The listing builds one solid part. Answer for the finished solid, in the listing's coordinates (mm). A direction names the side the tool comes from. Coordinates: 2 decimals unless noted, no trailing zeros. Loops run counter-clockwise (first coordinate to the right, second up) from the corner with the lowest first, then second, coordinate; pieces in that order, holes last. Notation, with made-up numbers: (-20.5, -37) -> (-10.5, -37) arc R21 cw to (-10.5, -5) -> close; hole circle Ø4 at (67, 53.25). An arc over 180 degrees is marked (long way). Answer in a Markdown table with one row per item.
```python
from build123d import *

# Parameters (mm, degrees)
F1_DEPTH  = 50.8
F2_T      = -1.5875
F4_DEPTH  = 1.5875
F5_W      = 15.875
F5_H      = 12.7
F6_DEPTH  = 1.5875
F7_W      = 1.5875
F7_H      = 12.7
F8_DEPTH  = 15.875
F10_D     = 6.7564
F11_W     = 15.875
F11_H     = 12.7
F12_DEPTH = 1.5875
F13_W     = 1.5875
F13_H     = 12.7
F14_DEPTH = 15.875
F16_D     = 6.7564


with BuildPart() as f1:
    # F0 (on Front) → F1 (new body)
    with BuildSketch(Plane.XZ):
        Polygon((-38.1, 114.3), (-76.2, 76.2), (-76.2, -76.2), (-38.1, -114.3), (0, -114.3), (38.1, -114.3), (76.2, -76.2), (76.2, 76.2), (38.1, 114.3), (0, 114.3), align=None)
    extrude(amount=F1_DEPTH)

    # F2
    f2_openings = [f1.faces().sort_by_distance(p)[0] for p in [
        (0, -50.8, 0),
    ]]
    offset(amount=F2_T, openings=f2_openings)

    # F3 (on face) → F4 (join)
    with BuildSketch(Plane.XZ.offset(50.8)):
        Polygon((-47.625, -85.725), (-76.2, -57.15), (-76.2, -76.2), (-38.1, -114.3), (38.1, -114.3), (76.2, -76.2), (76.2, -57.15), (47.204726897, -85.725), align=None)
    extrude(amount=F4_DEPTH)

    # F5 (on face) → F6 (join)
    with BuildSketch(Plane(origin=(-76.2, 0, 0), x_dir=(0, -1, 0), z_dir=(-1, 0, 0))):
        with Locations((42.8625, 50.8)):
            Rectangle(F5_W, F5_H)
    extrude(amount=F6_DEPTH)

    # F7 (on face) → F8 (join)
    with BuildSketch(Plane(origin=(-77.7875, 0, 0), x_dir=(0, -1, 0), z_dir=(-1, 0, 0))):
        with Locations((50.00625, 50.8)):
            Rectangle(F7_W, F7_H)
    extrude(amount=F8_DEPTH)

    # F10 (through all)
    with Locations(Plane(origin=(0, -49.2125, 0), x_dir=(-1, 0, 0), z_dir=(0, 1, 0))):
        with Locations((88.9, 50.8)):
            Hole(F10_D / 2)

    # F11 (on face) → F12 (join)
    with BuildSketch(Plane.YZ.offset(76.2)):
        with Locations((-42.8625, 50.8)):
            Rectangle(F11_W, F11_H)
    extrude(amount=F12_DEPTH)

    # F13 (on face) → F14 (join)
    with BuildSketch(Plane.YZ.offset(77.7875)):
        with Locations((-50.00625, 50.8)):
            Rectangle(F13_W, F13_H)
    extrude(amount=F14_DEPTH)

    # F16 (through all)
    with Locations(Plane(origin=(0, -49.2125, 0), x_dir=(-1, 0, 0), z_dir=(0, 1, 0))):
        with Locations((-88.9, 50.8)):
            Hole(F16_D / 2)


solid = f1.part
```
Item 1: Find the intervals of material crossed by probe 1 along Z at (x, y) = (-88.9, -49.7); probe 2 along Y at (x, z) = (51.5, -83); probe 3 along X at (y, z) = (-3, 22), in increasing order.
Findings below:
| item | result |
|---|---|
| probe 1 | z = 44.45 to 47.42, 54.18 to 57.15 |
| probe 2 | y = -52.39 to -50.8, -1.59 to 0 |
| probe 3 | x = -76.2 to -74.61, 74.61 to 76.2 |
Item 2: Flat-ended cylindrical pins translate along their axes: pin 1 Ø10 at (x, y) = (-64, -28.5) entering from -Z; pin 2 Ø10 at (y, z) = (-38.5, 84.5) entering from +X; pin 3 Ø1.3 at (x, z) = (77, 52.5) entering from +Y (3 decimals). Find the tip coordinate at first contact, or state that the pin passes through.
Findings below:
| item | result |
|---|---|
| pin 1 | stops at z = -93.4 |
| pin 2 | stops at x = 72.9 |
| pin 3 | stops at y = -34.925 |
Item 3: Determine the mould class of faces 6 (the face through (-1, -52.387, -92)), 7 (the face through (81, -49.4, 57.15)), 8 (the face through (55.767, -25.849, -94.388)), 9 (the face through (-1, -26, -112.712)) for opening direction Z: +Z half, -Z half, draft (parallel to the pull), parting line (faces both ways), or undercut.
Findings below:
| item | result |
|---|---|
| face 6 | draft |
| face 7 | +Z half |
| face 8 | undercut |
| face 9 | undercut |
Item 4: A cutting plane is placed at A-A, the plane x = -88.9. Determine the outline of the cut face in (y, z).
Findings below:
| item | result |
|---|---|
| outline | (-50.8, 44.45) -> (-49.21, 44.45) -> (-49.21, 47.42) -> (-50.8, 47.42) -> close; (-50.8, 54.18) -> (-49.21, 54.18) -> (-49.21, 57.15) -> (-50.8, 57.15) -> close |
Item 5: A cutting plane is placed at C-C, the plane y = -19.5. Determine the outline of the cut face in (x, z).
Findings below:
| item | result |
|---|---|
| outline | (-76.2, -76.2) -> (-38.1, -114.3) -> (38.1, -114.3) -> (76.2, -76.2) -> (76.2, 76.2) -> (38.1, 114.3) -> (-38.1, 114.3) -> (-76.2, 76.2) -> close; hole (-74.61, -75.54) -> (-37.44, -112.71) -> (37.44, -112.71) -> (74.61, -75.54) -> (74.61, 75.54) -> (37.44, 112.71) -> (-37.44, 112.71) -> (-74.61, 75.54) -> close |
Item 6: A tool of negligible diameter and unlimited length cuts with its end or side. For faces 1 (the face through (-55.767, -25.849, 94.388)), 2 (the face through (61.905, -51.583, -71.237)), 3 (the face through (77.788, -42, 51)), 4 (the face through (-84, -49.212, 51)), 5 (the face through (-56.288, -25.849, -93.867)), from which of +Z, -Z, +X, -X, +Y, -Y can it reach the whole face along a straight path? Write none if from no direction.
Findings below:
| item | result |
|---|---|
| face 1 | -Y |
| face 2 | +Z, -Y |
| face 3 | +Z, -Z, +X, +Y |
| face 4 | +Z, -Z, -X, +Y |
| face 5 | none |
Item 7: A cutting plane is placed at D-D, the plane x = -25. Determine the outline of the cut face in (y, z) (1 decimal), plus the area to 3 significant figures.
Findings below:
| item | result |
|---|---|
| outline | (-52.4, -114.3) -> (0, -114.3) -> (0, 114.3) -> (-50.8, 114.3) -> (-50.8, 112.7) -> (-1.6, 112.7) -> (-1.6, -112.7) -> (-50.8, -112.7) -> (-50.8, -85.7) -> (-52.4, -85.7) -> close |
| area | 565 mm2 |
Item 8: A cutting plane is placed at B-B, the plane z = 50.8. Determine the outline of the cut face in (x, y) (1 decimal), plus the area to 3 significant figures.
Findings below:
| item | result |
|---|---|
| outline | (-93.7, -50.8) -> (-92.3, -50.8) -> (-92.3, -49.2) -> (-93.7, -49.2) -> close; (-85.5, -50.8) -> (-74.6, -50.8) -> (-74.6, -1.6) -> (74.6, -1.6) -> (74.6, -50.8) -> (85.5, -50.8) -> (85.5, -49.2) -> (77.8, -49.2) -> (77.8, -34.9) -> (76.2, -34.9) -> (76.2, 0) -> (-76.2, 0) -> (-76.2, -34.9) -> (-77.8, -34.9) -> (-77.8, -49.2) -> (-85.5, -49.2) -> close; (92.3, -50.8) -> (93.7, -50.8) -> (93.7, -49.2) -> (92.3, -49.2) -> close |
| area | 478 mm2 |
